Source: three-view drawing plus pictorial views. Frame: mm from the lowest corner of the part. A direction names the side the tool comes from. Coordinates: 2 decimals unless noted, no trailing zeros. Write each loop counter-clockwise with the first axis right and the second up, starting at its lowest first coordinate (ties: lowest second). Pieces come first, ordered by that corner, then holes. Notation, with made-up numbers: (-8, 33) - (8, 33) arc R29 cw to (8, 70) - close; hole circle Ø4 at (-6.5, -6.5). An arc over 180 degrees is marked (long way). Put each result on its own line as item: value. Start each with the question number.
1. Cut plane A-A, the plane y = 15.25. Count the separate pieces of the cut face and the enclosed holes in it, and give its area (3 significant figures).
2. Pin query (flat end, axial travel): pin 1 (1.6 mm diameter, centred on x = 1.5, y = 11, fed in from -Z); pin 2 (3 mm diameter, centred on y = 10.5, z = 36, fed in from -X) (3 decimals); pin 3 (3.5 mm diameter, centred on x = 1.69, y = 5.25, fed in from +Z). Return the tip coordinate at first contact, or that it passes through.
3. Cut plane D-D, the plane z = 16.5. Return loops of the section in (x, y) (1 decimal), and give its area (3 significant figures).
4. Access query for the marked faces 1, 2, 3, 4 and 5. Directions: +Z, -Z, +X, -X, +Y, -Y. A direction counts if a zero-diameter tool reaches every point of the face in a straight line with its end or side. Return the directions, or none.
5. Line query: line 1 (X direction, y = 16, z = 27) (1 decimal); line 2 (Z direction, x = 5, y = 9.5). Output: solid intervals per line, ascending.
6. Cut plane C-C, the plane x = 48. Return loops of the section in (y, z).
7. Cut plane B-B, the plane y = 18.5. Return loops of the section in (x, z) (1 decimal), and give its area (3 significant figures).
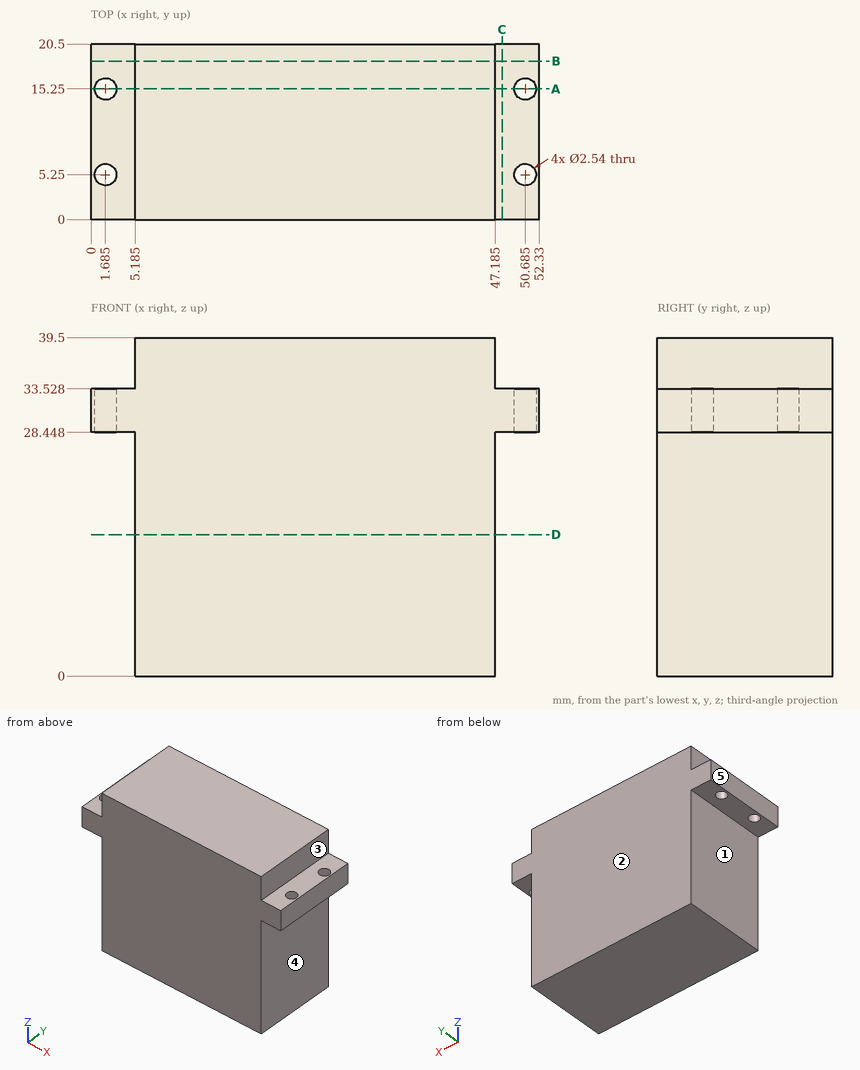
Report:
1. separate pieces: 3
1. enclosed holes: 0
1. area: 1,690 mm^2
2. pin 1: stops at z = 28.45
2. pin 2: stops at x = 5.185
2. pin 3: stops at z = 33.53
3. outline: (5.2, 0) - (47.2, 0) - (47.2, 20.5) - (5.2, 20.5) - close
3. area: 861 mm^2
4. face 1: -Z, -X, +Y, -Y
4. face 2: +Z, -Z, +X, -X, +Y
4. face 3: +Z, +X, +Y, -Y
4. face 4: -Z, +X, +Y, -Y
4. face 5: +Z, -Z, -X, +Y, -Y
5. line 1: x = 5.2 to 47.2
5. line 2: z = 28.45 to 33.53
6. outline: (0, 28.45) - (20.5, 28.45) - (20.5, 33.53) - (0, 33.53) - close
7. outline: (0, 28.4) - (5.2, 28.4) - (5.2, 0) - (47.2, 0) - (47.2, 28.4) - (52.3, 28.4) - (52.3, 33.5) - (47.2, 33.5) - (47.2, 39.5) - (5.2, 39.5) - (5.2, 33.5) - (0, 33.5) - close
7. area: 1,710 mm^2
